```python
from build123d import *

# Parameters (mm, degrees)
EXTRUDE_1_DEPTH     = 4.5
SKETCH_10_W         = 77.2
SKETCH_10_H         = 41.2
CUT_EXTRUDE_5_DEPTH = 79.027238834
SKETCH_16_R         = 1.6
CUT_EXTRUDE_6_DEPTH = 10
SKETCH_17_R         = 1.1
CUT_EXTRUDE_7_DEPTH = 10
FILLET_1_R          = 0.5


with BuildPart() as part:
    # 草图1 → 凸台-拉伸1 (new body)
    with BuildSketch(Plane(origin=(0, 0, 0), x_dir=(1, 0, 0), z_dir=(0, 1, 0))):
        Polygon((-58, -39), (-58, -52), (-52.25, -52), (-52.25, -39), (-28.75, -39), (-28.75, -52), (-23, -52), (-23, -39), (23, -39), (23, -52), (28.75, -52), (28.75, -39), (52.25, -39), (52.25, -52), (58, -52), (58, -39), (58, 39), (58, 52), (52.25, 52), (52.25, 39), (28.75, 39), (28.75, 52), (23, 52), (23, 39), (-23, 39), (-23, 52), (-28.75, 52), (-28.75, 39), (-52.25, 39), (-52.25, 52), (-58, 52), (-58, 39), align=None)
    extrude(amount=-EXTRUDE_1_DEPTH)

    # 草图10 → 切除-拉伸5 (cut, through all)
    with BuildSketch(Plane(origin=(0, 0, 0), x_dir=(1, 0, 0), z_dir=(0, 1, 0))):
        Rectangle(SKETCH_10_W, SKETCH_10_H)
    extrude(amount=-CUT_EXTRUDE_5_DEPTH, mode=Mode.SUBTRACT)

    # 草图16 → 切除-拉伸6 (cut)
    with BuildSketch(Plane(origin=(0, 0, 0), x_dir=(1, 0, 0), z_dir=(0, 1, 0))):
        with Locations(Location((19, 25.05, 0), (0, 0, 270))):
            Circle(SKETCH_16_R)
        with Locations(Location((49, 25.05, 0), (0, 0, 270))):
            Circle(SKETCH_16_R)
        with Locations(Location((-49, 25.05, 0), (0, 0, 90))):
            Circle(SKETCH_16_R)
        with Locations(Location((-19, 25.05, 0), (0, 0, 90))):
            Circle(SKETCH_16_R)
        with Locations(Location((49, -25.05, 0), (0, 0, 90))):
            Circle(SKETCH_16_R)
        with Locations(Location((19, -25.05, 0), (0, 0, 90))):
            Circle(SKETCH_16_R)
        with Locations(Location((-19, -25.05, 0), (0, 0, 270))):
            Circle(SKETCH_16_R)
        with Locations(Location((-49, -25.05, 0), (0, 0, 270))):
            Circle(SKETCH_16_R)
        with BuildLine():
            Line((-10, 26.3), (10, 26.3))
            ThreePointArc((10, 26.3), (11.25, 25.05), (10, 23.8))
            Line((10, 23.8), (-10, 23.8))
            ThreePointArc((-10, 23.8), (-11.25, 25.05), (-10, 26.3))
        make_face()
        with BuildLine():
            Line((-10, -26.3), (10, -26.3))
            ThreePointArc((10, -26.3), (11.25, -25.05), (10, -23.8))
            Line((10, -23.8), (-10, -23.8))
            ThreePointArc((-10, -23.8), (-11.25, -25.05), (-10, -26.3))
        make_face()
    extrude(amount=-CUT_EXTRUDE_6_DEPTH, mode=Mode.SUBTRACT)

    # 草图17 → 切除-拉伸7 (cut)
    with BuildSketch(Plane(origin=(0, 0, 0), x_dir=(1, 0, 0), z_dir=(0, 1, 0))):
        with Locations(Location((-54.5, -45.5, 0), (0, 0, 270))):
            Circle(SKETCH_17_R)
        with Locations(Location((-26.5, -45.5, 0), (0, 0, 270))):
            Circle(SKETCH_17_R)
        with Locations(Location((26.5, -45.5, 0), (0, 0, 90))):
            Circle(SKETCH_17_R)
        with Locations(Location((54.5, -45.5, 0), (0, 0, 90))):
            Circle(SKETCH_17_R)
        with Locations(Location((54.5, 45.5, 0), (0, 0, 270))):
            Circle(SKETCH_17_R)
        with Locations(Location((-26.5, 45.5, 0), (0, 0, 90))):
            Circle(SKETCH_17_R)
        with Locations(Location((-54.5, 45.5, 0), (0, 0, 90))):
            Circle(SKETCH_17_R)
        with Locations(Location((26.5, 45.5, 0), (0, 0, 270))):
            Circle(SKETCH_17_R)
    extrude(amount=-CUT_EXTRUDE_7_DEPTH, mode=Mode.SUBTRACT)

    # 圆角1
    fillet_1_edges = [part.edges().sort_by_distance(p)[0] for p in [
        (58, -2.25, 52),
        (52.25, -2.25, 52),
        (52.25, -2.25, 39),
        (28.75, -2.25, 39),
        (28.75, -2.25, 52),
        (23, -2.25, 52),
        (23, -2.25, 39),
        (-23, -2.25, 39),
        (-23, -2.25, 52),
        (-28.75, -2.25, 52),
        (-28.75, -2.25, 39),
        (-52.25, -2.25, 39),
        (-52.25, -2.25, 52),
        (-58, -2.25, 52),
        (-58, -2.25, -52),
        (-52.25, -2.25, -52),
        (-52.25, -2.25, -39),
        (-28.75, -2.25, -39),
        (-28.75, -2.25, -52),
        (-23, -2.25, -52),
        (-23, -2.25, -39),
        (23, -2.25, -39),
        (23, -2.25, -52),
        (28.75, -2.25, -52),
        (28.75, -2.25, -39),
        (52.25, -2.25, -39),
        (52.25, -2.25, -52),
        (58, -2.25, -52),
        (-38.6, -2.25, 20.6),
        (-38.6, -2.25, -20.6),
        (38.6, -2.25, -20.6),
        (38.6, -2.25, 20.6),
    ]]
    fillet(fillet_1_edges, radius=FILLET_1_R)


solid = part.part
```
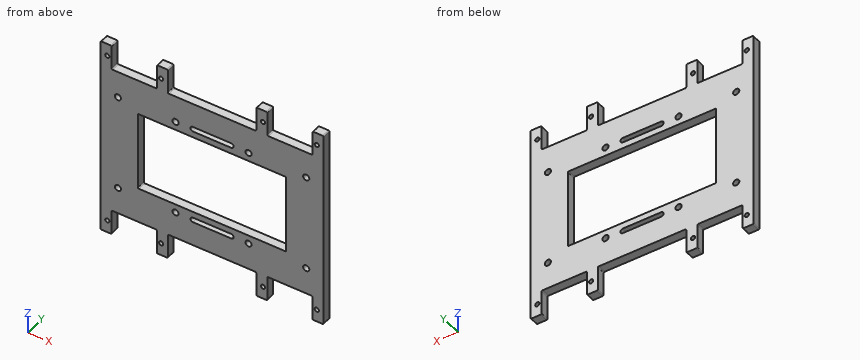
CAD build for the part. Positions are in the model's coordinates, mm. Coordinates: 2 decimals unless noted, no trailing zeros. Write each loop counter-clockwise with the first axis right and the second up, starting at its lowest first coordinate (ties: lowest second). Pieces come first, ordered by that corner, then holes. Notation, with made-up numbers: (-31, 54.25) -> (-16, 54.25) arc R24 ccw to (-16, 82.25) -> close; hole circle Ø10 at (-22, 72). An arc over 180 degrees is marked (long way). Use CSV: the item, a comma, the result in double quotes. Start each with the question number.
Item 1: Band-saw the part on C-C, the plane x = -49. Write the cut outline in (y, z), plus the area to 3 significant figures.
Item 2: Drop flat-ended pins along their axis: P1, Ø2, axis at x = 40.5, y = -3, coming from the -Z side; P2, Ø2, axis at x = -54.5, z = -45.5, coming from the -Y side; P3, Ø1.3, axis at x = 7, y = -2, coming from the +Z side. Give the stop position or say it passes through.
Item 3: Band-saw the part on A-A, the plane x = -34.5. Write the cut outline in (y, z).
Item 4: Band-saw the part on D-D, the plane x = 19. Write the cut outline in (y, z).
Item 5: Band-saw the part on B-B, the plane z = 14. Write the cut outline in (x, y).
Item 6: Wall check: probe 1 along X at (y, z) = (-1.65, -25.05); probe 2 along X at (y, z) = (-3.15, -47); probe 3 along Z at (x, y) = (-10, -4.05). Give the ranges that are in metal, low to high.
Response values:
1,outline,"(-4.5, -39) -> (0, -39) -> (0, -26.65) -> (-4.5, -26.65) -> close; (-4.5, -23.45) -> (0, -23.45) -> (0, 23.45) -> (-4.5, 23.45) -> close; (-4.5, 26.65) -> (0, 26.65) -> (0, 39) -> (-4.5, 39) -> close"
1,area,"322 mm2"
2,P1,"stops at z = -39"
2,P2,"passes through"
2,P3,"stops at z = 39"
3,outline,"(-4.5, -39) -> (0, -39) -> (0, -20.6) -> (-4.5, -20.6) -> close; (-4.5, 20.6) -> (0, 20.6) -> (0, 39) -> (-4.5, 39) -> close"
4,outline,"(-4.5, -39) -> (0, -39) -> (0, -26.65) -> (-4.5, -26.65) -> close; (-4.5, -23.45) -> (0, -23.45) -> (0, -20.6) -> (-4.5, -20.6) -> close; (-4.5, 20.6) -> (0, 20.6) -> (0, 23.45) -> (-4.5, 23.45) -> close; (-4.5, 26.65) -> (0, 26.65) -> (0, 39) -> (-4.5, 39) -> close"
5,outline,"(-58, -4.5) -> (-38.6, -4.5) -> (-38.6, 0) -> (-58, 0) -> close; (38.6, -4.5) -> (58, -4.5) -> (58, 0) -> (38.6, 0) -> close"
6,probe 1,"x = -58 to -50.6, -47.4 to -20.6, -17.4 to -11.25, 11.25 to 17.4, 20.6 to 47.4, 50.6 to 58"
6,probe 2,"x = -58 to -52.25, -28.75 to -23, 23 to 28.75, 52.25 to 58"
6,probe 3,"z = -39 to -26.3, -23.8 to -20.6, 20.6 to 23.8, 26.3 to 39"
